For this review, take the finished solid that the model builds, in its own axes (mm). A direction names the side the tool comes from. Coordinates: 2 decimals unless noted, no trailing zeros. Write each loop counter-clockwise with the first axis right and the second up, starting at its lowest first coordinate (ties: lowest second). Pieces come first, ordered by that corner, then holes. Notation, with made-up numbers: M -31.75,68.5 L -22.75,68.5 A20 cw -22.75,97.5 Z; hole C 75,35.5 d10. An arc over 180 degrees is marked long. Return JSON: item names as keys, results as strings.
```python
from build123d import *

# Parameters (mm, degrees)
F0_W     = 38.1
F0_H     = 50.8
F1_DEPTH = 9.525
F3_DEPTH = 9.526
F4_R     = 3.175
F5_DEPTH = 15.875
F6_R     = 3.175
F7_DEPTH = 9.526
F8_R     = 3.175
F9_DEPTH = 15.875


with BuildPart() as f1:
    # F0 (on Top) → F1 (new body)
    with BuildSketch(Plane.XY):
        Rectangle(F0_W, F0_H)
    extrude(amount=F1_DEPTH)

    # F2 (on face) → F3 (cut, through all)
    with BuildSketch(Plane.XY.offset(9.525)):
        with BuildLine():
            Line((-15.875, 15.875), (-19.05, 15.875))
            Line((-19.05, 15.875), (-19.05, -15.875))
            Line((-19.05, -15.875), (-15.875, -15.875))
            ThreePointArc((-15.875, -15.875), (-11.384872, -14.015128), (-9.525, -9.525))
            Line((-9.525, -9.525), (-9.525, 9.525))
            ThreePointArc((-9.525, 9.525), (-11.384872, 14.015128), (-15.875, 15.875))
        make_face()
        with BuildLine():
            Line((19.05, 15.875), (15.875, 15.875))
            ThreePointArc((15.875, 15.875), (11.384872, 14.015128), (9.525, 9.525))
            Line((9.525, 9.525), (9.525, -9.525))
            ThreePointArc((9.525, -9.525), (11.384872, -14.015128), (15.875, -15.875))
            Line((15.875, -15.875), (19.05, -15.875))
            Line((19.05, -15.875), (19.05, 15.875))
        make_face()
    extrude(amount=-F3_DEPTH, mode=Mode.SUBTRACT)

    # F4 (on face) → F5 (cut)
    with BuildSketch(Plane(origin=(-19.05, 0, 0), x_dir=(0, -1, 0), z_dir=(-1, 0, 0))):
        with Locations((-20.6375, 4.7625)):
            Circle(F4_R)
        with Locations((20.6375, 4.7625)):
            Circle(F4_R)
    extrude(amount=-F5_DEPTH, mode=Mode.SUBTRACT)

    # F6 (on face) → F7 (cut, through all)
    with BuildSketch(Plane.XY.offset(9.525)):
        Circle(F6_R)
    extrude(amount=-F7_DEPTH, mode=Mode.SUBTRACT)

    # F8 (on face) → F9 (cut)
    with BuildSketch(Plane.YZ.offset(19.05)):
        with Locations((-20.6375, 4.7625)):
            Circle(F8_R)
        with Locations((20.6375, 4.7625)):
            Circle(F8_R)
    extrude(amount=-F9_DEPTH, mode=Mode.SUBTRACT)


solid = f1.part
```
1. Clearance check with flat-ended pins moving along their axes: pin 1 Ø5 at (y, z) = (0.5, 6) entering from -X (3 decimals); pin 2 Ø4 at (y, z) = (-20.64, 4.76) entering from -X (3 decimals); pin 3 Ø1.9 at (y, z) = (19, 3.5) entering from +X (3 decimals); pin 4 Ø5 at (x, y) = (0, 0) entering from -Z. State where each tip first meets the part, or that it passes through.
Checks:
{"pin 1": "x = -9.525", "pin 2": "x = -3.175", "pin 3": "x = 3.175", "pin 4": "through"}
2. We need section A-A (y = 0). State the section outline as (x, z) points (3 decimals), plus the area to 3 significant figures.
Checks:
{"outline": "M -9.525,0 L -3.175,0 L -3.175,9.525 L -9.525,9.525 Z; M 3.175,0 L 9.525,0 L 9.525,9.525 L 3.175,9.525 Z", "area": "121 mm2"}
3. We need section B-B (x = 0). State the section outline as (y, z) points (3 decimals), plus the area to 3 significant figures.
Checks:
{"outline": "M -25.4,0 L -3.175,0 L -3.175,9.525 L -25.4,9.525 Z; M 3.175,0 L 25.4,0 L 25.4,9.525 L 3.175,9.525 Z", "area": "423 mm2"}
4. For faces 3 (the face through (3.175, 21, 5)), 4 (the face through (-3.175, -21, 5)), 5 (the face through (-11.34, 13.97, 4.83)), list the 3-axis set-ups (+Z, -Z, +X, -X, +Y, -Y) from which the entire face can be reached by the end or side of a thin tool; tool diameter is ignored.
Checks:
{"face 3": "+X", "face 4": "-X", "face 5": "+Z, -Z, -X"}
5. Wall thickness on L1, parallel to Y at x = 5.5, z = 3.5; L2, parallel to Y at x = 9, z = 3.75; L3, parallel to Z at x = -6, y = -20.5 (3 decimals): over which ranges is each line inside the solid? List them lowest first. Write a range as from..to.
Checks:
{"L1": "-25.4..-23.55, -17.72..17.72, 23.55..25.4", "L2": "-25.4..-23.65, -17.63..17.63, 23.65..25.4", "L3": "0..1.59, 7.935..9.525"}
6. We need section D-D (x = -14). Give the number of separate pieces and of enclosed holes in the cut face, plus the area to 3 significant figures.
Checks:
{"separate pieces": "2", "enclosed holes": "2", "area": "124 mm2"}
7. Draft analysis for pull direction Y (two halves, no side actions). For faces 1 (the face through (11.34, -13.97, 4.83)), 2 (the face through (4, 0, 9.525)), state which applies: +Y half, -Y half, draft (parallel to the pull), parting line (faces both ways), or undercut.
Checks:
{"face 1": "undercut", "face 2": "draft"}
